from build123d import *

# Parameters (mm, degrees)
SKETCH2_R               = 1.45
BOSS_EXTRUDE1_DEPTH     = 2.5
BOSS_EXTRUDE2_DEPTH     = 17.5
CUT_EXTRUDE1_DEPTH      = 38.148351242
CUT_EXTRUDE1_DEPTH_BACK = 38.148351242
SKETCH9_R               = 1.5
CUT_EXTRUDE2_DEPTH      = 38.43744783


with BuildPart() as part:
    # Sketch2 → Boss-Extrude1 (new body)
    with BuildSketch(Plane.XY):
        with BuildLine():
            Line((-3.75, 0), (-3.75, -1.75))
            ThreePointArc((-3.75, -1.75), (-4.335786438, -3.164213562), (-5.75, -3.75))
            Line((-5.75, -3.75), (-12.5, -3.75))
            ThreePointArc((-12.5, -3.75), (-13.785575219, -3.282088886), (-14.469615506, -2.097296355))
            Line((-14.469615506, -2.097296355), (-16.487605984, 9.347296355))
            ThreePointArc((-16.487605984, 9.347296355), (-17.171646271, 10.532088886), (-18.45722149, 11))
            Line((-18.45722149, 11), (-27, 11))
            ThreePointArc((-27, 11), (-27.707106781, 11.292893219), (-28, 12))
            Line((-28, 12), (-28, 14))
            Line((-28, 14), (28, 14))
            Line((28, 14), (28, 12))
            ThreePointArc((28, 12), (27.707106781, 11.292893219), (27, 11))
            Line((27, 11), (18.45722149, 11))
            ThreePointArc((18.45722149, 11), (17.171646271, 10.532088886), (16.487605984, 9.347296355))
            Line((16.487605984, 9.347296355), (14.469615506, -2.097296355))
            ThreePointArc((14.469615506, -2.097296355), (13.785575219, -3.282088886), (12.5, -3.75))
            Line((12.5, -3.75), (5.75, -3.75))
            ThreePointArc((5.75, -3.75), (4.335786438, -3.164213562), (3.75, -1.75))
            Line((3.75, -1.75), (3.75, 0))
            ThreePointArc((3.75, 0), (0, 3.75), (-3.75, 0))
        make_face()
        with Locations((-7.5, 0)):
            Circle(SKETCH2_R, mode=Mode.SUBTRACT)
        with Locations((7.5, 0)):
            Circle(SKETCH2_R, mode=Mode.SUBTRACT)
    extrude(amount=-BOSS_EXTRUDE1_DEPTH)

    # Sketch3 → Boss-Extrude2 (add)
    with BuildSketch(Plane(origin=(0, 0, -2.5), x_dir=(-1, 0, 0), z_dir=(0, 0, -1))):
        with BuildLine():
            Line((-11, -2.75), (-11, 6))
            ThreePointArc((-11, 6), (-9.535533906, 9.535533906), (-6, 11))
            Line((-6, 11), (6, 11))
            ThreePointArc((6, 11), (9.535533906, 9.535533906), (11, 6))
            Line((11, 6), (11, -2.75))
            ThreePointArc((11, -2.75), (11.292893219, -3.457106781), (12, -3.75))
            Line((12, -3.75), (12.5, -3.75))
            ThreePointArc((12.5, -3.75), (13.785575219, -3.282088886), (14.469615506, -2.097296355))
            Line((14.469615506, -2.097296355), (16.487605984, 9.347296355))
            ThreePointArc((16.487605984, 9.347296355), (17.171646271, 10.532088886), (18.45722149, 11))
            Line((18.45722149, 11), (27, 11))
            ThreePointArc((27, 11), (27.707106781, 11.292893219), (28, 12))
            Line((28, 12), (28, 14))
            Line((28, 14), (-28, 14))
            Line((-28, 14), (-28, 12))
            ThreePointArc((-28, 12), (-27.707106781, 11.292893219), (-27, 11))
            Line((-27, 11), (-18.45722149, 11))
            ThreePointArc((-18.45722149, 11), (-17.171646271, 10.532088886), (-16.487605984, 9.347296355))
            Line((-16.487605984, 9.347296355), (-14.469615506, -2.097296355))
            ThreePointArc((-14.469615506, -2.097296355), (-13.785575219, -3.282088886), (-12.5, -3.75))
            Line((-12.5, -3.75), (-12, -3.75))
            ThreePointArc((-12, -3.75), (-11.292893219, -3.457106781), (-11, -2.75))
        make_face()
    extrude(amount=BOSS_EXTRUDE2_DEPTH)

    # Sketch6 → Cut-Extrude1 (cut, two sides: drawn at the far end of the back side and taken through both)
    with BuildSketch(Plane(origin=(0, 0, 0), x_dir=(0, 0, -1), z_dir=(1, 0, 0)).offset(-CUT_EXTRUDE1_DEPTH_BACK)):
        Polygon((6, -3.75), (20, 11), (20, -3.75), align=None)
    extrude(amount=CUT_EXTRUDE1_DEPTH + CUT_EXTRUDE1_DEPTH_BACK, mode=Mode.SUBTRACT)

    # Sketch9 → Cut-Extrude2 (cut, through all)
    with BuildSketch(Plane.XZ.offset(-11)):
        with Locations((22.7, -15)):
            Circle(SKETCH9_R)
        with Locations((22.7, -5)):
            Circle(SKETCH9_R)
    cut_extrude2 = extrude(amount=-CUT_EXTRUDE2_DEPTH, mode=Mode.SUBTRACT)

    # Mirror1: Cut-Extrude2 across plane
    add(cut_extrude2.mirror(Plane(origin=(0, 0, 0), x_dir=(0, 0, 1), z_dir=(1, 0, 0))), mode=Mode.SUBTRACT)


solid = part.part
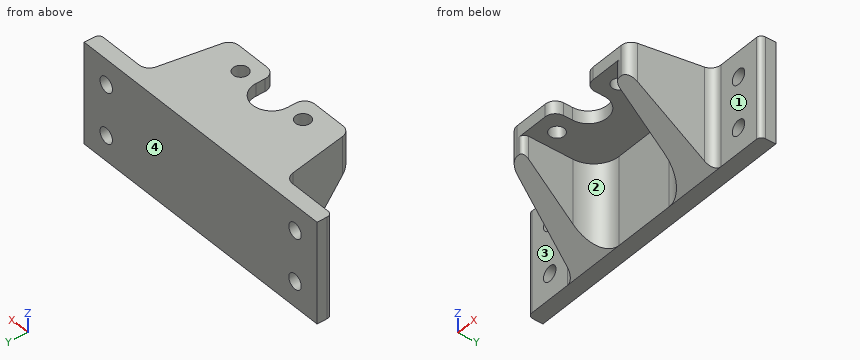
Can you work these out from the model? Positions are in its coordinate system, mm. Face numbers are marked on the shaded views. A direction names the side the tool comes from. Coordinates: 2 decimals unless noted, no trailing zeros. Loops run counter-clockwise (first coordinate to the right, second up) from the corner with the lowest first, then second, coordinate; pieces in that order, holes last. Notation, with made-up numbers: (-11, 49) - (-7, 49) arc R24 cw to (-7, 79) - close; hole circle Ø11 at (27.25, 17). An arc over 180 degrees is marked (long way). Put each result on its own line as item: value. Start each with the question number.
Item 1: For pin 1 (0.5 mm diameter, centred on y = -0.5, z = -1.5, fed in from -X); pin 2 (4 mm diameter, centred on y = 8.5, z = -14, fed in from -X); pin 3 (3.5 mm diameter, centred on x = 22.7, z = -15, fed in from -Y), each with a flat end and sliding along its axis, tell me the tip position at first contact or that it passes through.
Item 2: Suppose I cut it at B-B (z = -5). State how many separate pieces and enclosed holes the cut face has, and give its area (3 significant figures).
Item 3: Which directions (+Z, -Z, +X, -X, +Y, -Y) give clear straight access to the entire face, cutting with the end or side of a thin tool? Please do the marked faces 1, 2, 3 and 4.
Item 4: Suppose I cut it at D-D (y = 7.25). Please give me the cut outline in (x, z), and give its area (3 significant figures).
Item 5: Suppose I cut it at C-C (x = -7.5). Please give me the cut outline in (y, z), and give its area (3 significant figures).
Item 6: If I drill on line 1 along Z through (x, y) = (-22.7, 13.3); line 2 along Y through (x, z) = (-7.5, -1.9); line 3 along X through (y, z) = (10.25, -11.5), over which ranges is the centre line in solid material (lowest first)?
Item 7: Suppose I cut it at A-A (x = -22.7). Please give me the cut outline in (y, z), and give its area (3 significant figures).
Here are the results:
1. pin 1: x = -14.8
1. pin 2: x = -17.13
1. pin 3: y = 11
2. separate pieces: 3
2. enclosed holes: 0
2. area: 292 mm²
3. face 1: +Z, -Z, +X, -Y
3. face 2: -Z, -Y
3. face 3: +Z, -Z, -X, -Y
3. face 4: +Z, -Z, +X, -X, +Y
4. outline: (-16.12, -16.44) - (-10.84, -16.44) - (-10.84, -2.5) - (10.84, -2.5) - (10.84, -16.44) - (16.12, -16.44) - (16.12, 0) - (-16.12, 0) - close
4. area: 228 mm²
5. outline: (-3.75, -2.5) - (-1.45, -2.5) - (-1.45, 0) - (-3.75, 0) - close; (1.45, -2.5) - (10.77, -2.5) - (10.77, -19.78) - (11, -20) - (14, -20) - (14, 0) - (1.45, 0) - close
5. area: 93.6 mm²
6. line 1: -20 to -16.5, -13.5 to -6.5, -3.5 to 0
6. line 2: -3.75 to -1.45, 1.45 to 14
6. line 3: -16.9 to -8.63, 8.63 to 16.9
7. outline: (11, -20) - (14, -20) - (14, -16.5) - (11, -16.5) - close; (11, -13.5) - (14, -13.5) - (14, -6.5) - (11, -6.5) - close; (11, -3.5) - (14, -3.5) - (14, 0) - (11, 0) - close
7. area: 42.0 mm²
